Verification items for this drawing (mm, ordinates from the low corner). A direction names the side the tool comes from. Round coordinates to 2 decimals unless told otherwise and drop trailing zeros. Loops run counter-clockwise (first coordinate to the right, second up) from the corner with the lowest first, then second, coordinate; pieces in that order, holes last. Notation, with made-up numbers: (40.25, 79.5) -> (61.25, 79.5) arc R17 ccw to (61.25, 108.5) -> close; hole circle Ø11 at (87.5, 83.25). An arc over 180 degrees is marked (long way). Use a Markdown table: item, result. Add a question column.
Q1. Gauge pin test, flat ends, axial feed: P1, Ø5, axis at y = 5.5, z = 9.5, coming from the +X side; P2, Ø1, axis at y = 1.5, z = 7.5, coming from the +X side. Record the tip position at first contact, or that the pin passes through.
Q2. Set-up check for the marked faces 1 and 2: record each of +Z, -Z, +X, -X, +Y, -Y from which the full face is reachable in a straight line by a thin tool's end or side.
Q3. Sectioned sample at C-C, the plane x = 7.75. Enter the section's corners in (y, z).
Q4. Material ranges on L1, parallel to Y at x = 7.5, z = 10.5 (1 decimal); L2, parallel to X at y = 6.75, z = 1 (1 decimal); L3, parallel to Z at x = 1.25, y = 3.5, recorded low to high.
Q5. Sectioned sample at B-B, the plane y = 6.75. Enter the section's corners in (x, z).
Q6. Sectioned sample at A-A, the plane z = 4.75. Enter the section's corners in (x, y).
Q7. Release check for a two-part mould opening along X. For the marked faces 3, 4 and 5 record: released by +X, released by -X, zero draft, split by the parting line, or undercut.
Q8. Sectioned sample at D-D, the plane z = 7.5. Enter the section's corners in (x, y), then the cut area to 3 significant figures.
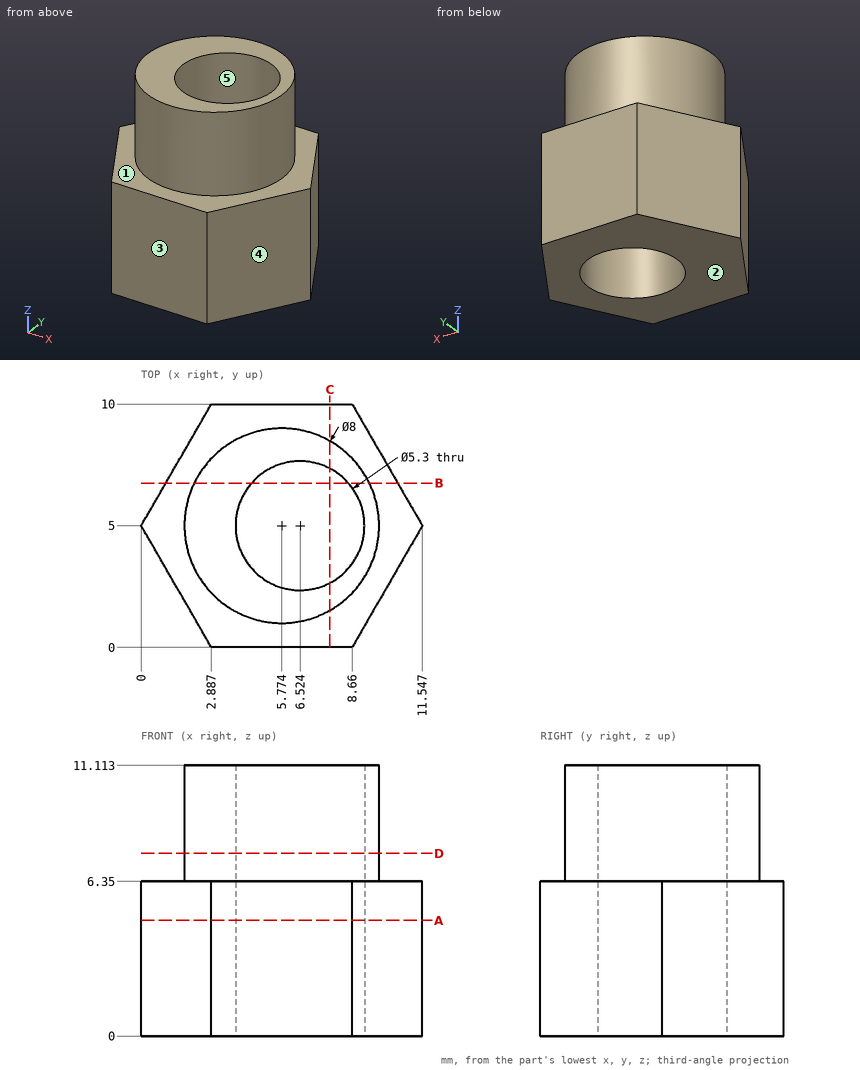
Values:
| question | item | result |
|---|---|---|
| 1 | P1 | x = 9.77 |
| 1 | P2 | x = 8.42 |
| 2 | face 1 | +Z |
| 2 | face 2 | -Z, +X, -X, +Y, -Y |
| 3 | outline | (0, 0) -> (2.65, 0) -> (2.65, 11.11) -> (1.52, 11.11) -> (1.52, 6.35) -> (0, 6.35) -> close; (7.35, 0) -> (10, 0) -> (10, 6.35) -> (8.48, 6.35) -> (8.48, 11.11) -> (7.35, 11.11) -> close |
| 4 | L1 | 1.4 to 2.5, 7.5 to 8.6 |
| 4 | L2 | 1 to 4.5, 8.5 to 10.5 |
| 4 | L3 | 0 to 6.35 |
| 5 | outline | (1.01, 0) -> (4.53, 0) -> (4.53, 11.11) -> (2.18, 11.11) -> (2.18, 6.35) -> (1.01, 6.35) -> close; (8.51, 0) -> (10.54, 0) -> (10.54, 6.35) -> (9.37, 6.35) -> (9.37, 11.11) -> (8.51, 11.11) -> close |
| 6 | outline | (0, 5) -> (2.89, 0) -> (8.66, 0) -> (11.55, 5) -> (8.66, 10) -> (2.89, 10) -> close; hole circle Ø5.3 at (6.52, 5) |
| 7 | face 3 | zero draft |
| 7 | face 4 | released by +X |
| 7 | face 5 | undercut |
| 8 | outline | circle Ø8 at (5.77, 5); hole circle Ø5.3 at (6.52, 5) |
| 8 | area | 28.2 mm^2 |
